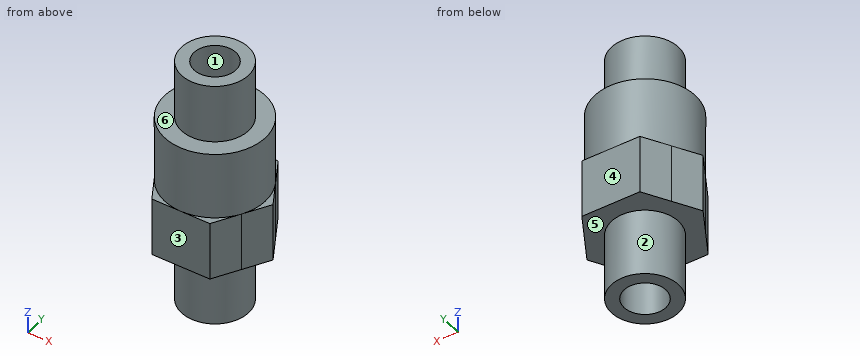
from build123d import *

# Parameters (mm, degrees)
SKETCH1_R           = 6
SKETCH1_R_2         = 4
BOSS_EXTRUDE1_DEPTH = 7
SKETCH1_3_R         = 4
SKETCH1_3_R_2       = 2.5
BOSS_EXTRUDE2_DEPTH = 15
BOSS_EXTRUDE3_START = 8
SKETCH1_4_R         = 6
SKETCH1_4_R_2       = 4
BOSS_EXTRUDE3_DEPTH = 8
BOSS_EXTRUDE4_START = 15
SKETCH1_5_R         = 4
SKETCH1_5_R_2       = 2.5
BOSS_EXTRUDE4_DEPTH = 15


with BuildPart() as part:
    # Sketch1 → Boss-Extrude1 (new body)
    # profile 1 of 7: a face of its own
    with BuildSketch(Plane.XY):
        with BuildLine():
            ThreePointArc((-5.196152514, 2.999999842), (-3.000000081, 5.196152376), (-3e-09, 6))
            Line((-3e-09, 6), (-3.464101615, 6))
            Line((-3.464101615, 6), (-5.196152514, 2.999999842))
        make_face()
    # profile 2 of 7: a face of its own
    with BuildSketch(Plane.XY):
        with BuildLine():
            ThreePointArc((-3e-09, 6), (3.000000209, 5.196152302), (5.196152666, 2.999999578))
            Line((5.196152666, 2.999999578), (3.464101615, 6))
            Line((3.464101615, 6), (-3e-09, 6))
        make_face()
    # profile 3 of 7: a face of its own
    with BuildSketch(Plane.XY):
        with BuildLine():
            Line((5.196152428, -2.999999991), (6.92820323, 0))
            Line((6.92820323, 0), (5.196152666, 2.999999578))
            ThreePointArc((5.196152666, 2.999999578), (5.795555021, 1.552914036), (6, 0))
            ThreePointArc((6, 0), (5.795554959, -1.552914265), (5.196152428, -2.999999991))
        make_face()
    # profile 4 of 7: a face of its own
    with BuildSketch(Plane.XY):
        with BuildLine():
            Line((3.464101615, -6), (5.196152428, -2.999999991))
            ThreePointArc((5.196152428, -2.999999991), (3.000000007, -5.196152419), (5e-09, -6))
            Line((5e-09, -6), (3.464101615, -6))
        make_face()
    # profile 5 of 7: a face of its own
    with BuildSketch(Plane.XY):
        with BuildLine():
            Line((-3.464101615, -6), (5e-09, -6))
            ThreePointArc((5e-09, -6), (-3.000000229, -5.19615229), (-5.19615269, -2.999999537))
            Line((-5.19615269, -2.999999537), (-3.464101615, -6))
        make_face()
    # profile 6 of 7: a face of its own
    with BuildSketch(Plane.XY):
        with BuildLine():
            ThreePointArc((-5.19615269, -2.999999537), (-6, 1.76e-07), (-5.196152514, 2.999999842))
            Line((-5.196152514, 2.999999842), (-6.92820323, 0))
            Line((-6.92820323, 0), (-5.19615269, -2.999999537))
        make_face()
    # profile 7 of 7: a face of its own
    with BuildSketch(Plane.XY):
        Circle(SKETCH1_R)
        Circle(SKETCH1_R_2, mode=Mode.SUBTRACT)
    extrude(amount=-BOSS_EXTRUDE1_DEPTH)

    # Sketch1_3 → Boss-Extrude2 (add)
    with BuildSketch(Plane.XY):
        Circle(SKETCH1_3_R)
        Circle(SKETCH1_3_R_2, mode=Mode.SUBTRACT)
    extrude(amount=-BOSS_EXTRUDE2_DEPTH)

    # Sketch1_4 → Boss-Extrude3 (add)
    with BuildSketch(Plane.XY.offset(BOSS_EXTRUDE3_START)):
        with Locations(Location((0, 0, 0), (0, 0, 150))):
            Circle(SKETCH1_4_R)
        Circle(SKETCH1_4_R_2, mode=Mode.SUBTRACT)
    extrude(amount=-BOSS_EXTRUDE3_DEPTH)

    # Sketch1_5 → Boss-Extrude4 (add)
    with BuildSketch(Plane.XY.offset(BOSS_EXTRUDE4_START)):
        Circle(SKETCH1_5_R)
        Circle(SKETCH1_5_R_2, mode=Mode.SUBTRACT)
    extrude(amount=-BOSS_EXTRUDE4_DEPTH)


solid = part.part
For this review, take the finished solid that the model builds, in its own axes (mm). Face numbers are marked on the shaded views. A direction names the side the tool comes from. Coordinates: 2 decimals unless noted, no trailing zeros. Loops run counter-clockwise (first coordinate to the right, second up) from the corner with the lowest first, then second, coordinate; pieces in that order, holes last. Notation, with made-up numbers: (51.25, -21.5) - (102.25, -21.5) arc R22 cw to (102.25, 6.5) - close; hole circle Ø4 at (75.5, 1). An arc over 180 degrees is marked (long way). Use a Markdown table: item, result. Add a question column.
Item 1: Insertion check: pin 1 Ø0.9 at (x, y) = (-6.5, -0.5) entering from +Z; pin 2 Ø1.5 at (x, y) = (3, -4) entering from -Z; pin 3 Ø6 at (y, z) = (-3.5, -11) entering from -X; pin 4 Ø3 at (x, y) = (0, 0) entering from +Z. Each pin has a flat end and moves straight along its axis. Give the tip position at first contact, or say it passes through.
Item 2: We need section C-C (y = 4.5). Give the boundary of the cut face in (x, z).
Item 3: For line 1 (Y direction, x = 0, z = -3); line 2 (Y direction, x = 0, z = 8.5); line 3 (X direction, y = 1.5, z = -2.75), list the stretches that pass through material, from the lowest coordinate up.
Item 4: We need section B-B (y = -2). Give the boundary of the cut face in (x, z), and give its area (3 significant figures).
Item 5: Mouldability with a two-part tool opening along X and no side actions: class the marked faces 1, 2 and 3 as pulls with the +X half, pulls with the -X half, needs draft (parallel to the pull), parting line crosses it, or undercut.
Item 6: Tool access review of the marked faces 4, 5 and 6: name each direction out of +Z, -Z, +X, -X, +Y, -Y from which nothing blocks a thin tool from reaching the whole face with its end or side.
Item 7: We need section A-A (z = -5.75). Give the boundary of the cut face in (x, y).
Item 8: We need section D-D (z = 0.5). Give the boundary of the cut face in (x, y).
Results list:
| question | item | result |
|---|---|---|
| 1 | pin 1 | stops at z = 0 |
| 1 | pin 2 | stops at z = -7 |
| 1 | pin 3 | stops at x = -3.97 |
| 1 | pin 4 | passes through |
| 2 | outline | (-4.33, -7) - (4.33, -7) - (4.33, 0) - (3.97, 0) - (3.97, 8) - (-3.97, 8) - (-3.97, 0) - (-4.33, 0) - close |
| 3 | line 1 | y = -6 to -2.5, 2.5 to 6 |
| 3 | line 2 | y = -4 to -2.5, 2.5 to 4 |
| 3 | line 3 | x = -6.06 to -2, 2 to 6.06 |
| 4 | outline | (-5.77, -7) - (-3.46, -7) - (-3.46, -15) - (-1.5, -15) - (-1.5, 15) - (-3.46, 15) - (-3.46, 8) - (-5.66, 8) - (-5.66, 0) - (-5.77, 0) - close; (1.5, -15) - (3.46, -15) - (3.46, -7) - (5.77, -7) - (5.77, 0) - (5.66, 0) - (5.66, 8) - (3.46, 8) - (3.46, 15) - (1.5, 15) - close |
| 4 | area | 185 mm^2 |
| 5 | face 1 | undercut |
| 5 | face 2 | parting line crosses it |
| 5 | face 3 | needs draft |
| 6 | face 4 | +Z, -Z, +X, -X, +Y |
| 6 | face 5 | -Z |
| 6 | face 6 | +Z |
| 7 | outline | (-6.93, 0) - (-3.46, -6) - (3.46, -6) - (6.93, 0) - (3.46, 6) - (-3.46, 6) - close; hole circle Ø5 at (0, 0) |
| 8 | outline | circle Ø12 at (0, 0); hole circle Ø5 at (0, 0) |
